Geometry: final body of the model. Coordinates: model frame, mm. Face numbers are marked on the shaded views. A direction names the side the tool comes from. Coordinates: 2 decimals unless noted, no trailing zeros. Write each loop counter-clockwise with the first axis right and the second up, starting at its lowest first coordinate (ties: lowest second). Pieces come first, ordered by that corner, then holes. Notation, with made-up numbers: (62.25, 16) - (108.25, 16) arc R14 ccw to (108.25, 34) - close; hole circle Ø10 at (50.5, -19). An arc over 180 degrees is marked (long way). Answer as a JSON object with one key per item and string values. Group by question number.
Item 1: First-contact query: pin 1 Ø2.5 at (x, y) = (2, 41.74) entering from -Z; pin 2 Ø1.8 at (x, y) = (2, 41.74) entering from -Z; pin 3 Ø6 at (x, y) = (9.5, 34) entering from +Z; pin 4 Ø1.4 at (y, z) = (41.5, 30) entering from +X. Flat tips, straight axial feed; report the tip coordinate or a pass-through.
Item 2: Line query: line 1 along Y through (x, z) = (2, 38.35); line 2 along Z through (x, y) = (2.25, 40.5); line 3 along X through (y, z) = (21.5, 36). Output: solid intervals per line, ascending. Write a range as from..to.
Item 3: Section C-C on x = 2. State how many separate pieces and enclosed holes the cut face has, and give its area (3 significant figures).
Item 4: Section B-B on z = 52.5. Return loops of the section in (x, y).
Item 5: Mould query, pull axis Y, two halves, no side actions, for the marked faces 1 and 2. Classes: pulls with the +Y half, pulls with the -Y half, needs draft (parallel to the pull), parting line crosses it, or undercut.
Item 6: Section D-D on z = 40.5. Return loops of the section in (x, y).
Item 7: Section A-A on y = 29. Return loops of the section in (x, z).
Item 8: Set-up query: the marked faces 3 and 4. Return all of +Z, -Z, +X, -X, +Y, -Y with unobstructed straight access to the full face (end or side cutting, diameter ignored); none if empty.
```python
from build123d import *

# Parameters (mm, degrees)
F0_W      = 28
F0_H      = 60
F1_DEPTH  = 4
F2_W      = 4
F2_H      = 5
F3_DEPTH  = 3
F4_W      = 4
F4_H      = 5
F5_DEPTH  = 4
F6_R      = 1
F7_DEPTH  = 25
F8_R      = 10
F9_W      = 8
F9_H      = 6
F9_R      = 1
F9_W_2    = 11
F9_H_2    = 3
F10_DEPTH = 25
F12_DEPTH = 7.5
F13_SIZE  = 7


with BuildPart() as f1:
    # F0 (on Right) → F1 (new body)
    with BuildSketch(Plane.YZ):
        with Locations((25.744221, 41.653179)):
            Rectangle(F0_W, F0_H)
    extrude(amount=F1_DEPTH)

    # F2 (on face) → F3 (join)
    with BuildSketch(Plane.YZ.offset(4)):
        with Locations((21.744221, 44.153179)):
            Rectangle(F2_W, F2_H)
        with Locations((20.744221, 14.153179)):
            Rectangle(F2_W, F2_H)
    extrude(amount=F3_DEPTH)

    # F4 (on face) → F5 (join)
    with BuildSketch(Plane(origin=(0, 0, 0), x_dir=(0, -1, 0), z_dir=(-1, 0, 0))):
        with Locations((-41.744221, 38.653179)):
            Rectangle(F4_W, F4_H)
        with Locations((-41.744221, 28.653179)):
            Rectangle(F4_W, F4_H)
        with Locations((-41.744221, 18.653179)):
            Rectangle(F4_W, F4_H)
    extrude(amount=-F5_DEPTH)

    # F6 (on face) → F7 (cut)
    with BuildSketch(Plane.XY.offset(41.153179)):
        with Locations((2, 41.744221)):
            Circle(F6_R)
        Polygon((4, 43.744221), (2.828427, 43.744221), (4, 42.572648), align=None)
    extrude(amount=-F7_DEPTH, mode=Mode.SUBTRACT)

    # F8
    f8_edges = [f1.edges().sort_by_distance(p)[0] for p in [
        (2, 11.744221, 71.653179),
    ]]
    fillet(f8_edges, radius=F8_R)

    # F9 (on face) → F10 (cut)
    with BuildSketch(Plane(origin=(0, 0, 0), x_dir=(0, -1, 0), z_dir=(-1, 0, 0))):
        with Locations((-31.244221, 63.153179)):
            Rectangle(F9_W, F9_H)
        with Locations((-31.244221, 63.153179)):
            Circle(F9_R, mode=Mode.SUBTRACT)
        with Locations((-31.244221, 63.153179)):
            Circle(F9_R)
        with Locations((-31.244221, 53.153179)):
            Rectangle(F9_W_2, F9_H_2)
    extrude(amount=-F10_DEPTH, mode=Mode.SUBTRACT)

    # F11 (on face) → F12 (join)
    with BuildSketch(Plane.YZ.offset(4)):
        Polygon((39.744221, 41.153179), (39.744221, 51.653179), (36.744221, 51.653179), (31.744221, 51.653179), (31.744221, 18.653179), (39.744221, 18.653179), (39.744221, 21.153179), (39.744221, 26.153179), (39.744221, 31.153179), (39.744221, 36.153179), align=None)
    extrude(amount=F12_DEPTH)

    # F13
    f13_edges = [f1.edges().sort_by_distance(p)[0] for p in [
        (11.5, 31.744221, 35.153179),
    ]]
    chamfer(f13_edges, length=F13_SIZE)


solid = f1.part
```
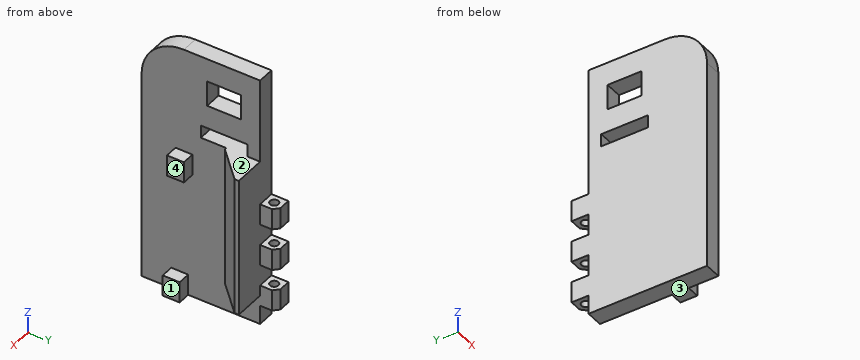
Checks:
{
 "1": {"pin 1": "z = 16.15", "pin 2": "through", "pin 3": "z = 51.65", "pin 4": "x = 4"},
 "2": {"line 1": "11.74..40.74, 42.74..43.74", "line 2": "16.15..21.15, 26.15..31.15, 36.15..41.15", "line 3": "0..4"},
 "3": {"separate pieces": "4", "enclosed holes": "2", "area": "1,610 mm^2"},
 "4": {"outline": "(0, 11.74) - (4, 11.74) - (4, 25.74) - (0, 25.74) - close; (0, 36.74) - (4, 36.74) - (4, 39.74) - (0, 39.74) - close"},
 "5": {"face 1": "needs draft", "face 2": "undercut"},
 "6": {"outline": "(0, 11.74) - (4, 11.74) - (4, 31.74) - (4.5, 31.74) - (11.5, 38.74) - (11.5, 39.74) - (4, 39.74) - (4, 42.57) - (2.83, 43.74) - (0, 43.74) - close; hole circle Ø2 at (2, 41.74)"},
 "7": {"outline": "(0, 11.65) - (4, 11.65) - (4, 51.65) - (0, 51.65) - close; (0, 54.65) - (4, 54.65) - (4, 60.15) - (0, 60.15) - close; (0, 66.15) - (4, 66.15) - (4, 71.65) - (0, 71.65) - close"},
 "8": {"face 3": "-Z, +X, -X, +Y, -Y", "face 4": "+Z, -Z, +X, -Y"}
}
